Build history of the part. All positions in model axes, mm. A direction names the side the tool comes from. Coordinates: 2 decimals unless noted, no trailing zeros. Loops run counter-clockwise (first coordinate to the right, second up) from the corner with the lowest first, then second, coordinate; pieces in that order, holes last.
Item 1: Mould opens along Z. For faces 1 (the face through (-0.794, 13.875, 6.044)), 2 (the face through (-4.1, 0, 2.3)), 3 (the face through (1, 3.556, -2)) say: released by +Z, released by -Z, zero draft, split by the parting line, or undercut.
Item 2: Cut at A-A (z = -1.5). List the corners of the cut face in (x, y), and give its area (3 significant figures).
Item 3: Flat gauge pins, fed straight in: pin 1 (1 mm diameter, centred on y = 14, z = -0.5, fed in from +X); pin 2 (1 mm diameter, centred on x = -7, y = 3, fed in from +Z); pin 3 (1.5 mm diameter, centred on x = -6, y = 5.5, fed in from +Z). Where does each tip first touch, or does it go through?
Item 4: Cut at D-D (x = -4.25). List the corners of the cut face in (y, z).
Item 5: Cut at C-C (y = 12). List the corners of the cut face in (x, z).
Item 6: Cut at B-B (x = 0). List the corners of the cut face in (y, z) (3 decimals), and give its area (3 significant figures).
Item 7: 3-axis set-ups, long thin cutter, end or side, ignore diameter. For faces 4 (the face through (-3.93, 1.75, 2.08)), 5 (the face through (2, 6.35, -6)), 6 (the face through (3, 21.193, 0)): which of +Z, -Z, +X, -X, +Y, -Y reach the whole face in a straight line?
Item 8: Drill centre lines: line 1 along Z through (x, y) = (0, 7.75); line 2 along Y through (x, z) = (6.5, -6.5); line 3 along Y through (x, z) = (4, -1.5). Where is each one in solid material? Low to high.
from build123d import *

# Parameters (mm, degrees)
F_8_32_TAPPED_HOLE1_D = 4.1656
CUT_EXTRUDE1_DEPTH    = 3.556


with BuildPart() as part:
    # Sketch3 → Revolve1 (revolve)
    with BuildSketch(Plane.XY):
        Polygon((0, 0), (9.525, 0), (9.525, 6.35), (6.096, 6.35), (6.096, 21.193), (0, 21.193), align=None)
    revolve(axis=Axis((0, 21.193, 0), (0, -1, 0)))

    # #8-32 Tapped Hole1 (through all)
    with Locations(Plane(origin=(0, 21.193, 0), x_dir=(1, 0, 0), z_dir=(0, 1, 0))):
        with Locations((0, 0)):
            Hole(F_8_32_TAPPED_HOLE1_D / 2)

    # Sketch6 → Cut-Extrude1 (cut)
    with BuildSketch(Plane.XZ):
        Polygon((2.369915953, 4.552749906), (-2.757839099, 4.328782373), (-5.127755052, -0.223967533), (-2.369915953, -4.552749906), (2.757839099, -4.328782373), (5.127755052, 0.223967533), align=None)
    extrude(amount=-CUT_EXTRUDE1_DEPTH, mode=Mode.SUBTRACT)


solid = part.part
Filled sheet:
1. face 1: split by the parting line
1. face 2: zero draft
1. face 3: undercut
2. outline: (-9.41, 0) - (-4.31, 0) - (-4.31, 3.56) - (-1.45, 3.56) - (-1.45, 21.19) - (-5.91, 21.19) - (-5.91, 6.35) - (-9.41, 6.35) - close; (1.45, 3.56) - (4.23, 3.56) - (4.23, 0) - (9.41, 0) - (9.41, 6.35) - (5.91, 6.35) - (5.91, 21.19) - (1.45, 21.19) - close
2. area: 214 mm2
3. pin 1: stops at x = 6.1
3. pin 2: stops at z = 6.96
3. pin 3: stops at z = 7.95
4. outline: (0, -8.52) - (6.35, -8.52) - (6.35, -4.37) - (21.19, -4.37) - (21.19, 4.37) - (6.35, 4.37) - (6.35, 8.52) - (0, 8.52) - (0, 1.46) - (3.56, 1.46) - (3.56, -1.6) - (0, -1.6) - close
5. outline: circle Ø12.19 at (0, 0); hole circle Ø4.17 at (0, 0)
6. outline: (0, -9.525) - (6.35, -9.525) - (6.35, -6.096) - (21.193, -6.096) - (21.193, -2.083) - (3.556, -2.083) - (3.556, -4.449) - (0, -4.449) - close; (0, 4.449) - (3.556, 4.449) - (3.556, 2.083) - (21.193, 2.083) - (21.193, 6.096) - (6.35, 6.096) - (6.35, 9.525) - (0, 9.525) - close
6. area: 197 mm2
7. face 4: -Y
7. face 5: +Y
7. face 6: +Z, -Z, +X, -X, +Y
8. line 1: z = -6.1 to -2.08, 2.08 to 6.1
8. line 2: y = 0 to 6.35
8. line 3: y = 3.56 to 21.19
